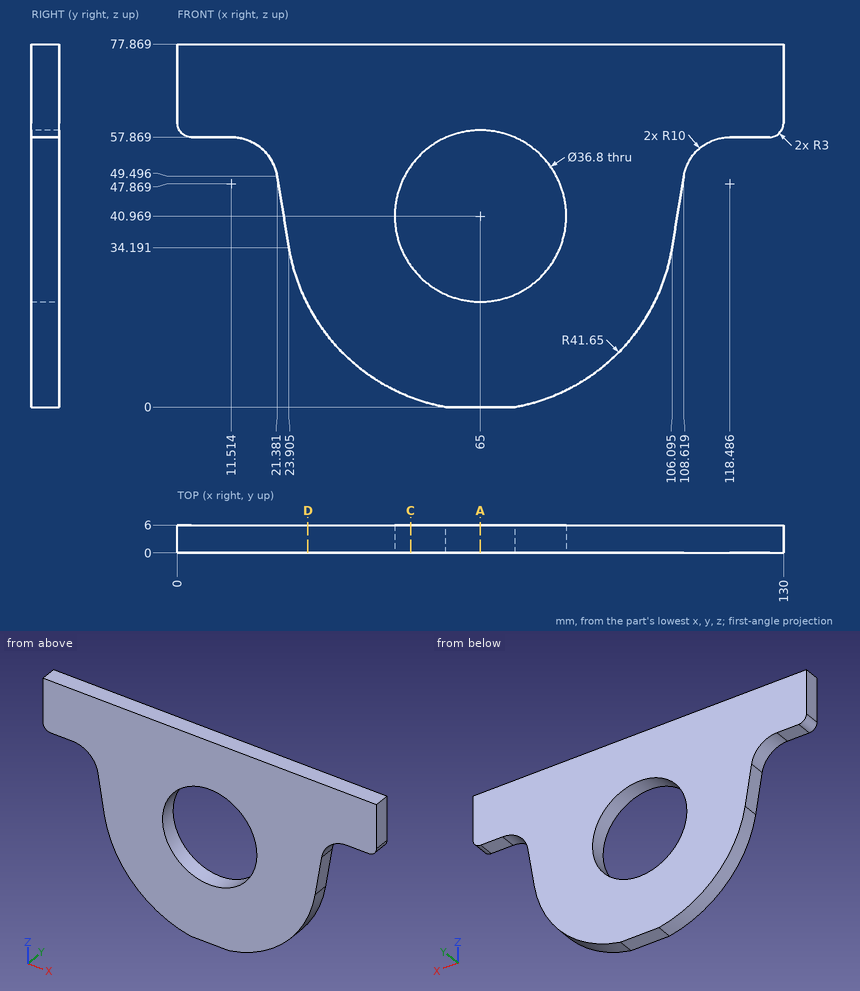
For this review, use the dimensioned drawing (mm, ordinates from the lowest corner) and the shaded views. Round coordinates to 2 decimals unless told otherwise and drop trailing zeros. Order: outer loops, then holes, each group sorted by start corner. A loop starts at its lowest first (then second) coordinate and runs counter-clockwise, first axis right, second up. Notation, with made-up numbers: M 82,-7 L 105,-7 A22 cw 105,5 Z; hole C 78.5,78 d10. An arc over 180 degrees is marked long. Use a Markdown table: item, result.
1) Consider section C-C (x = 50). Write out the cut boundary in (y, z) (1 decimal).
Report:
| item | result |
|---|---|
| outline | M 0,2.1 L 6,2.1 L 6,30.3 L 0,30.3 Z; M 0,51.6 L 6,51.6 L 6,77.9 L 0,77.9 Z |
2) Wall thickness on line 1 along Z through (x, y) = (64.5, 4.55) (1 decimal); line 2 along Z through (x, y) = (123, 3); line 3 along X through (y, z) = (5.05, 31.5) (1 decimal): over which ranges is each line inside the solid? List them lowest first. Write a range as [from, to].
Report:
| item | result |
|---|---|
| line 1 | [0, 22.6], [59.4, 77.9] |
| line 2 | [57.87, 77.87] |
| line 3 | [24.4, 49.2], [80.8, 105.6] |
3) Consider section A-A (x = 65). Write out the cut boundary in (y, z).
Report:
| item | result |
|---|---|
| outline | M 0,0 L 6,0 L 6,22.57 L 0,22.57 Z; M 0,59.37 L 6,59.37 L 6,77.87 L 0,77.87 Z |
4) Insertion check: pin 1 (2 mm diameter, centred on y = 0.5, z = 26, fed in from +X); pin 2 (2 mm diameter, centred on x = 101.5, y = 4.5, fed in from -Z) (1 decimal); pin 3 (2 mm diameter, centred on x = 31, y = 3, fed in from -Z). Each pin has a flat end and moves straight along its axis. Give the tip position at first contact, or say it passes through.
Report:
| item | result |
|---|---|
| pin 1 | x = 104.24 |
| pin 2 | z = 19.2 |
| pin 3 | z = 15.56 |
5) Consider section D-D (x = 28). Write out the cut boundary in (y, z) (1 decimal).
Report:
| item | result |
|---|---|
| outline | M 0,21.8 L 6,21.8 L 6,77.9 L 0,77.9 Z |
